Here's the drawing with two shaded views (mm, measured from the low corner). I have some questions. A direction names the side the tool comes from. Round coordinates to 2 decimals unless told otherwise and drop trailing zeros. Loops run counter-clockwise (first coordinate to the right, second up) from the corner with the lowest first, then second, coordinate; pieces in that order, holes last.
(1) I want a section at B-B on x = 111. Write out the boundary of the cut face in (y, z) (1 decimal), plus the area to 3 significant figures.
(2) I want a section at A-A on z = 107.5. Write out the boundary of the cut face in (x, y), plus the area to 3 significant figures.
(3) Will these pins go through, and if not, where does the flat tip stop? pin 1 Ø8 at (x, z) = (127, 55.5) entering from +Y; pin 2 Ø7.5 at (y, z) = (104.5, 77) entering from -X; pin 3 Ø3 at (x, z) = (84.5, 24.5) entering from -Y; pin 4 Ø1.5 at (y, z) = (57, 56.5) entering from +X.
(4) I want a section at C-C on z = 75. Write out the boundary of the cut face in (x, y).
(5) I want a section at D-D on y = 100. Write out the boundary of the cut face in (x, z).
(6) If I drill on line 1 along Y through (x, z) = (37, 105.5); line 2 along X through (y, z) = (8, 42.5); line 3 along Y through (x, z) = (112, 84), over which ranges is the centre line in solid material (lowest first)?
(7) Thinking about a two-plate mould opening in Y: for the marked faces 4, 5, 6 and 7, which applies, released by +Y, released by -Y, zero draft, split by the parting line, or undercut?
(8) Which directions (+Z, -Z, +X, -X, +Y, -Y) give clear straight access to the entire face, cutting with the end or side of a thin tool? Please do the marked faces 1, 2 and 3.
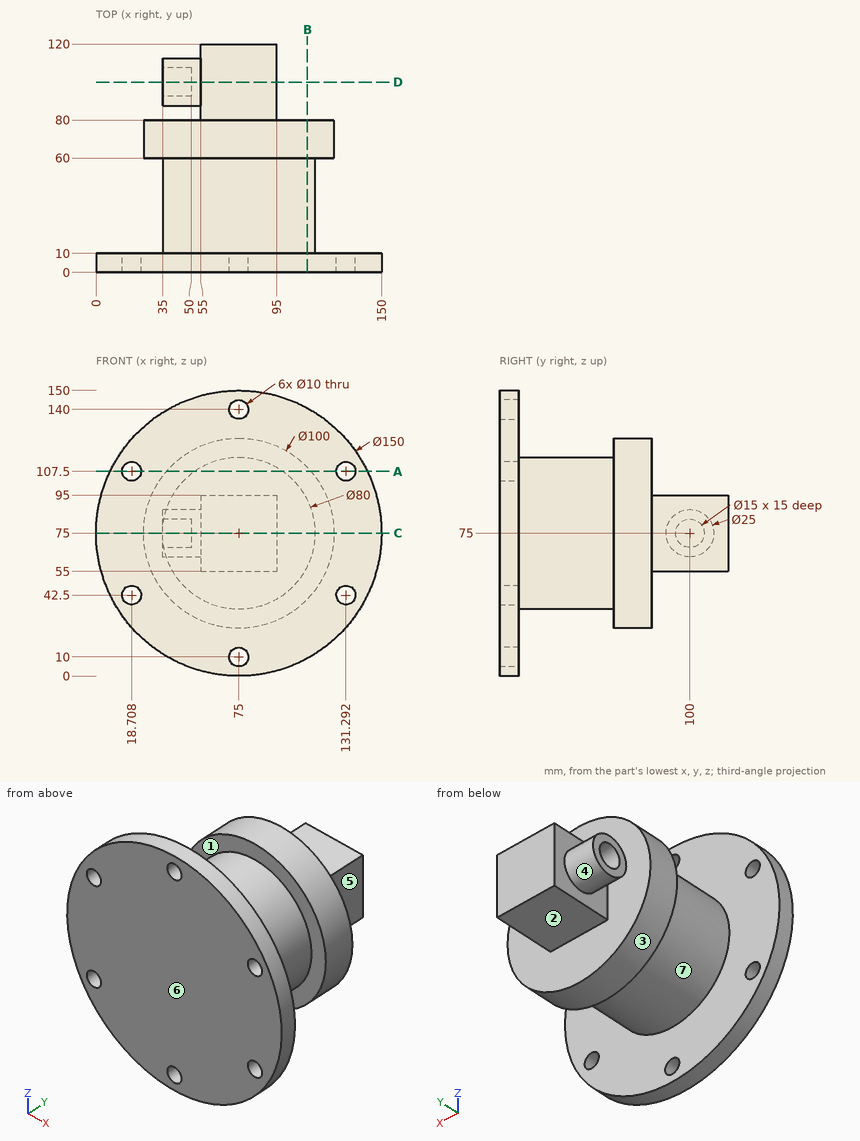
Filled sheet:
1. outline: (0, 9.2) - (10, 9.2) - (10, 57.6) - (60, 57.6) - (60, 40.3) - (80, 40.3) - (80, 109.7) - (60, 109.7) - (60, 92.4) - (10, 92.4) - (10, 140.8) - (0, 140.8) - close
1. area: 4,450 mm2
2. outline: (7.41, 0) - (13.71, 0) - (13.71, 10) - (7.41, 10) - close; (23.71, 0) - (126.29, 0) - (126.29, 10) - (98.32, 10) - (98.32, 60) - (113, 60) - (113, 80) - (37, 80) - (37, 60) - (51.68, 60) - (51.68, 10) - (23.71, 10) - close; (136.29, 0) - (142.59, 0) - (142.59, 10) - (136.29, 10) - close
2. area: 5,000 mm2
3. pin 1: stops at y = 10
3. pin 2: stops at x = 35
3. pin 3: stops at y = 0
3. pin 4: stops at x = 110.85
4. outline: (0, 0) - (150, 0) - (150, 10) - (115, 10) - (115, 60) - (125, 60) - (125, 80) - (95, 80) - (95, 120) - (55, 120) - (55, 112.5) - (35, 112.5) - (35, 107.5) - (50, 107.5) - (50, 92.5) - (35, 92.5) - (35, 87.5) - (55, 87.5) - (55, 80) - (25, 80) - (25, 60) - (35, 60) - (35, 10) - (0, 10) - close
5. outline: (35, 62.5) - (55, 62.5) - (55, 55) - (95, 55) - (95, 95) - (55, 95) - (55, 87.5) - (35, 87.5) - (35, 82.5) - (50, 82.5) - (50, 67.5) - (35, 67.5) - close
6. line 1: y = 0 to 10, 60 to 80
6. line 2: x = 7.41 to 13.71, 23.71 to 126.29, 136.29 to 142.59
6. line 3: y = 0 to 80
7. face 4: undercut
7. face 5: zero draft
7. face 6: released by -Y
7. face 7: undercut
8. face 1: none
8. face 2: -Z, +X, -X, +Y
8. face 3: +Y
